Design review of the part shown in the three views and the two pictorial views. Dimensions are in mm from the part's minimum x, y and z. Coordinates: 2 decimals unless noted, no trailing zeros. Loops run counter-clockwise (first coordinate to the right, second up) from the corner with the lowest first, then second, coordinate; pieces in that order, holes last. Notation, with made-up numbers: (-26.5, 67) -> (31.5, 67) arc R16 cw to (31.5, 89) -> close; hole circle Ø3 at (-36, 85). An arc over 180 degrees is marked (long way). Answer in a Markdown table with one row per item.
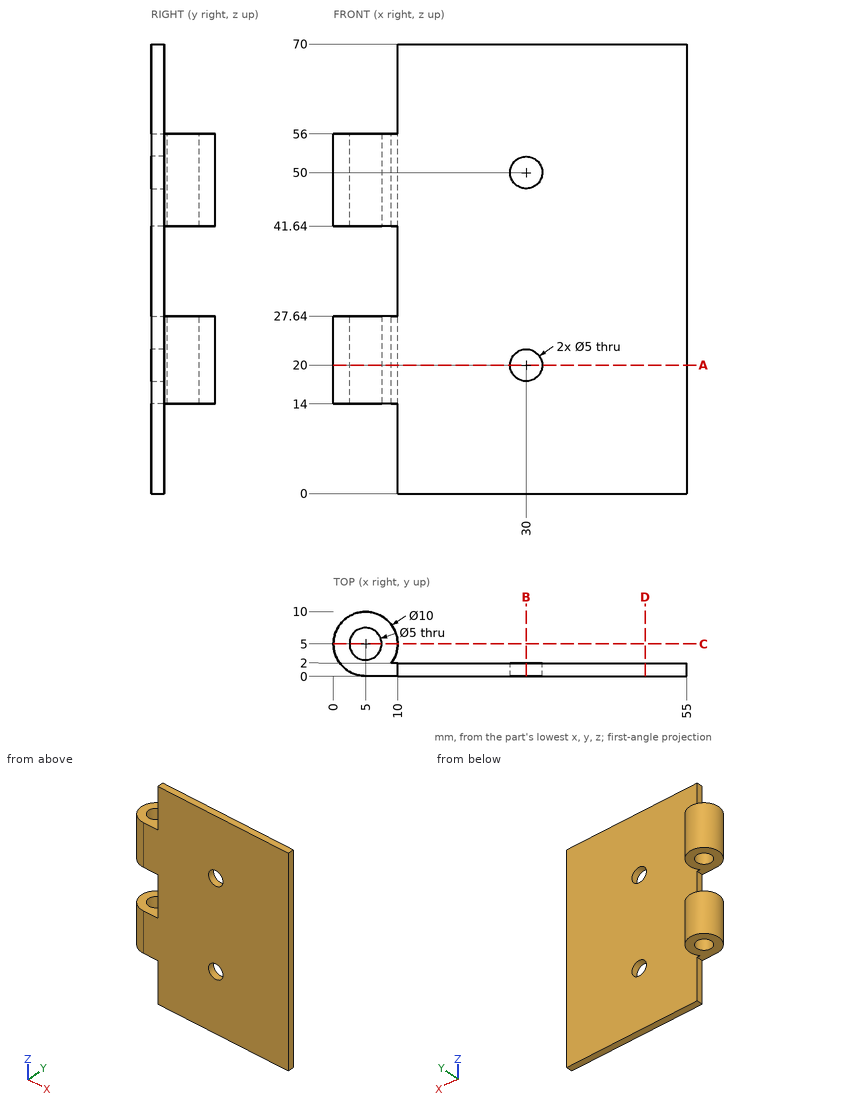
Item 1: Take a section at C-C, the plane y = 5. State the section outline as (x, z) points, and give its area (3 significant figures).
Worked answers:
| item | result |
|---|---|
| outline | (0, 14) -> (2.5, 14) -> (2.5, 27.64) -> (0, 27.64) -> close; (0, 41.64) -> (2.5, 41.64) -> (2.5, 56) -> (0, 56) -> close; (7.5, 14) -> (10, 14) -> (10, 27.64) -> (7.5, 27.64) -> close; (7.5, 41.64) -> (10, 41.64) -> (10, 56) -> (7.5, 56) -> close |
| area | 140 mm² |
Item 2: Insertion check: pin 1 (5 mm diameter, centred on x = 5, y = 6.5, fed in from -Z); pin 2 (2 mm diameter, centred on y = 0.5, z = 33.5, fed in from -X); pin 3 (6 mm diameter, centred on x = 9, z = 22.5, fed in from -Y); pin 4 (3 mm diameter, centred on x = 30, z = 20, fed in from +Y). Each pin has a flat end and moves straight along its axis. Give the tip position at first contact, or say it passes through.
Worked answers:
| item | result |
|---|---|
| pin 1 | z = 14 |
| pin 2 | x = 10 |
| pin 3 | y = 0 |
| pin 4 | through |
Item 3: For L1, parallel to Y at x = 5, z = 22; L2, parallel to Z at x = 6, y = 2.5; L3, parallel to X at y = 0.5, z = 9.5, list the stretches that pass through material, from the lowest coordinate up.
Worked answers:
| item | result |
|---|---|
| L1 | 0 to 2.5, 7.5 to 10 |
| L2 | 14 to 27.64, 41.64 to 56 |
| L3 | 10 to 55 |
Item 4: Take a section at D-D, the plane x = 48.5. State the section outline as (y, z) points.
Worked answers:
| item | result |
|---|---|
| outline | (0, 0) -> (2, 0) -> (2, 70) -> (0, 70) -> close |
Item 5: Take a section at A-A, the plane z = 20. State the section outline as (x, y) points.
Worked answers:
| item | result |
|---|---|
| outline | (5, 0) -> (27.5, 0) -> (27.5, 2) -> (9, 2) arc R5 ccw (long way) to start; (32.5, 0) -> (55, 0) -> (55, 2) -> (32.5, 2) -> close; hole circle Ø5 at (5, 5) |
Item 6: Take a section at B-B, the plane x = 30. State the section outline as (y, z) points, and give its area (3 significant figures).
Worked answers:
| item | result |
|---|---|
| outline | (0, 0) -> (2, 0) -> (2, 17.5) -> (0, 17.5) -> close; (0, 22.5) -> (2, 22.5) -> (2, 47.5) -> (0, 47.5) -> close; (0, 52.5) -> (2, 52.5) -> (2, 70) -> (0, 70) -> close |
| area | 120 mm² |
